Check sheet for the modelled part. Datum: model origin and axes. Units: mm. Face numbers are marked on the shaded views. A direction names the side the tool comes from. Give positions to 0.01 mm unless a question says otherwise; leave off trailing zeros. Write each loop counter-clockwise with the first axis right and the second up, starting at its lowest first coordinate (ties: lowest second). Pieces come first, ordered by that corner, then holes. Notation, with made-up numbers: M 84,81.25 L 112,81.25 A23 ccw 112,104.25 Z; hole C 87.25,88.5 d7. An arc over 180 degrees is marked long. Write item = value, one per line. Start each with the question number.
1) Cross-section at A-A, the plane y = 54. Record the cut outline in (x, z), plus the area to 3 significant figures.
2) Mould release check, pull along X, two halves, no side actions. Record for the marked faces 3, 4 and 5: released by +X, released by -X, zero draft, split by the parting line, or undercut.
3) Go/stop test with flat-tipped pins: pin 1 (1 mm diameter, centred on x = -8.5, y = -5, fed in from -Z); pin 2 (2 mm diameter, centred on y = 10, z = 5, fed in from -X); pin 3 (1.5 mm diameter, centred on x = 8.5, z = 5, fed in from +Y); pin 4 (2 mm diameter, centred on y = 14.5, z = 2, fed in from +X). Record where each tip stops, or that it passes through.
4) Cross-section at B-B, the plane x = 4. Give the number of separate pieces and of enclosed holes in the cut face, plus the area to 3 significant figures.
5) Access from +Z, -Z, +X, -X, +Y, -Y to the whole of each face (thin tool, end or side, straight path). Record for the marked faces 1 and 2.
6) Cross-section at C-C, the plane z = 3.25. Record the cut outline in (x, y).
7) Scan lines: line 1 along Y through (x, z) = (-9, 1.5); line 2 along X through (y, z) = (51.5, 3.75); line 3 along X through (y, z) = (77, 3). Record each from-to range of solid material in increasing order. Write a range as [from, to].
8) Cross-section at D-D, the plane y = 81.5. Record the cut outline in (x, z).
```python
from build123d import *

# Parameters (mm, degrees)
SKETCH1_R           = 7.75
BOSS_EXTRUDE1_DEPTH = 7


with BuildPart() as part:
    # Sketch1 → Boss-Extrude1 (new body)
    with BuildSketch(Plane.XY):
        with BuildLine():
            Line((-14.121781939, 65.817369233), (-14.121781939, -52.520726978))
            ThreePointArc((-14.121781939, -52.520726978), (-1.121781939, -65.520726978), (11.878218061, -52.520726978))
            Line((11.878218061, -52.520726978), (11.878218061, 65.817369233))
            ThreePointArc((11.878218061, 65.817369233), (12.166002849, 69.197986251), (13.021075204, 72.481314255))
            ThreePointArc((13.021075204, 72.481314255), (-1.121781939, 92.479273022), (-15.264639082, 72.481314255))
            ThreePointArc((-15.264639082, 72.481314255), (-14.409566727, 69.197986251), (-14.121781939, 65.817369233))
        make_face()
        with Locations((-1.121781939, -52.520726978)):
            Circle(SKETCH1_R, mode=Mode.SUBTRACT)
        with Locations((-1.121781939, -22.520726978)):
            Circle(SKETCH1_R, mode=Mode.SUBTRACT)
        with Locations((-1.121781939, 77.479273022)):
            Circle(SKETCH1_R, mode=Mode.SUBTRACT)
        Polygon((-9.121781939, 3.957653989), (-9.121781939, -3.042346011), (6.878218061, -7.32953309), (6.878218061, 8.67046691), align=None, mode=Mode.SUBTRACT)
        Polygon((-9.121781939, 31.957653989), (6.878218061, 27.67046691), (6.878218061, 43.67046691), (-9.121781939, 38.957653989), align=None, mode=Mode.SUBTRACT)
        Polygon((6.878218061, 56.67046691), (-9.121781939, 60.957653989), (-9.121781939, 44.957653989), (6.878218061, 49.67046691), align=None, mode=Mode.SUBTRACT)
        Polygon((-9.121781939, 9.957653989), (6.878218061, 14.67046691), (6.878218061, 21.67046691), (-9.121781939, 25.957653989), align=None, mode=Mode.SUBTRACT)
    extrude(amount=BOSS_EXTRUDE1_DEPTH)


solid = part.part
```
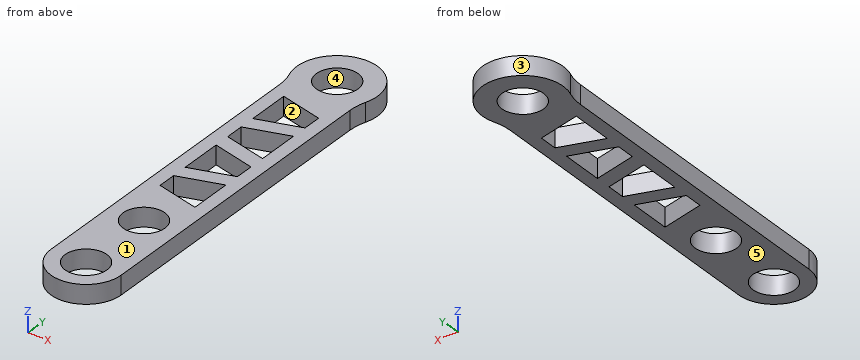
Reply:
q1.outline = M -14.12,0 L -9.12,0 L -9.12,7 L -14.12,7 Z; M 6.88,0 L 11.88,0 L 11.88,7 L 6.88,7 Z
q1.area = 70.0 mm2
q2.face_3 = split by the parting line
q2.face_4 = undercut
q2.face_5 = zero draft
q3.pin_1 = 0
q3.pin_2 = -14.12
q3.pin_3 = 89.57
q3.pin_4 = 11.88
q4.separate_pieces = 8
q4.enclosed_holes = 0
q4.area = 526 mm2
q5.face_1 = +Z, +X, -X, +Y, -Y
q5.face_2 = +Z, -Z
q6.outline = M -15.26,72.48 A20 cw -14.12,65.82 L -14.12,-52.52 A13 ccw 11.88,-52.52 L 11.88,65.82 A20 cw 13.02,72.48 A15 ccw long Z; hole M -9.12,-3.04 L 6.88,-7.33 L 6.88,8.67 L -9.12,3.96 Z; hole M -9.12,9.96 L 6.88,14.67 L 6.88,21.67 L -9.12,25.96 Z; hole M -9.12,31.96 L 6.88,27.67 L 6.88,43.67 L -9.12,38.96 Z; hole M -9.12,44.96 L 6.88,49.67 L 6.88,56.67 L -9.12,60.96 Z; hole C -1.12,-52.52 d15.5; hole C -1.12,-22.52 d15.5; hole C -1.12,77.48 d15.5
q7.line_1 = [-62.86, -3.07], [3.99, 9.99], [25.93, 31.93], [38.99, 44.99], [60.93, 90.24]
q7.line_2 = [-14.12, -9.12], [6.88, 11.88]
q7.line_3 = [-16.11, -8.86], [6.61, 13.87]
q8.outline = M -15.57,0 L -7.75,0 L -7.75,7 L -15.57,7 Z; M 5.5,0 L 13.33,0 L 13.33,7 L 5.5,7 Z
